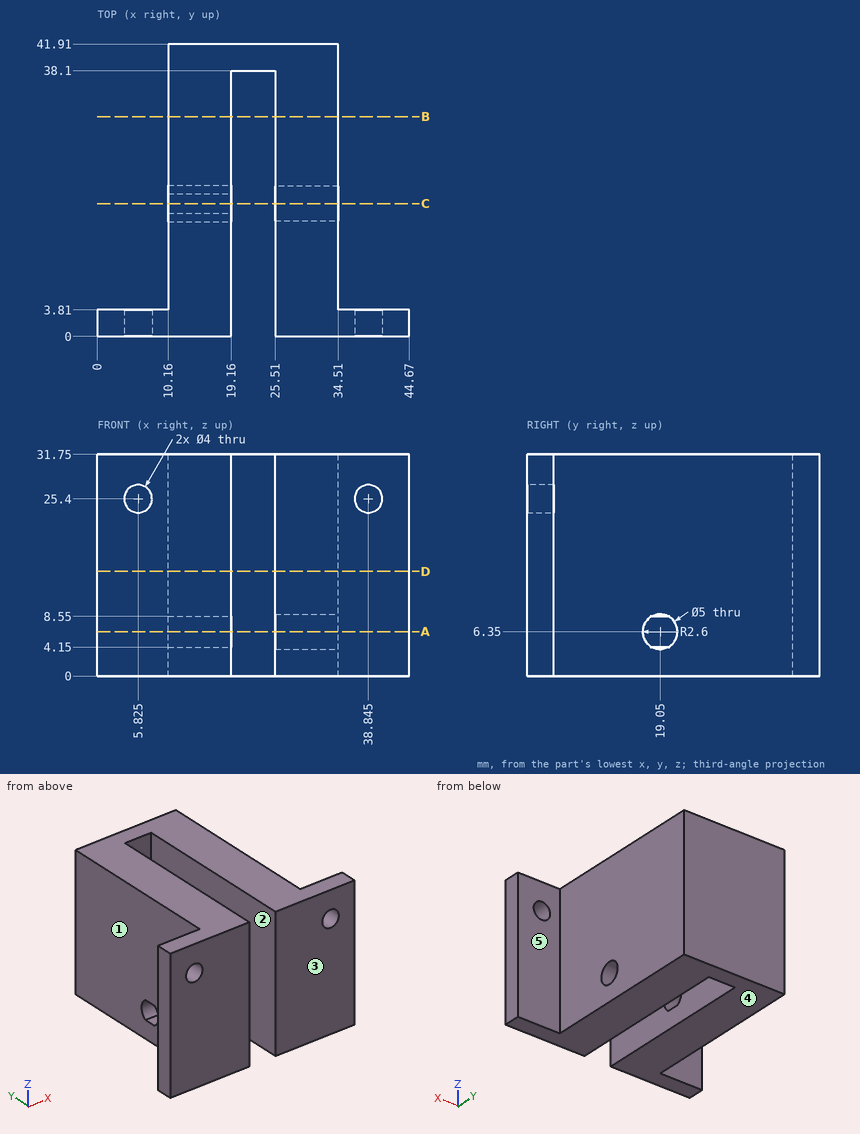
Check sheet for the drawn part. Datum: minimum x, y, z corner. Units: mm. A direction names the side the tool comes from. Round coordinates to 2 decimals unless told otherwise and drop trailing zeros. Loops run counter-clockwise (first coordinate to the right, second up) from the corner with the lowest first, then second, coordinate; pieces in that order, holes last. Notation, with made-up numbers: (2.5, 8) - (51.5, 8) arc R24 ccw to (51.5, 42) - close; hole circle Ø1 at (83.5, 16). An arc over 180 degrees is marked (long way). Write item = value, one per line. Start each with the question number.
1. Section check D-D on z = 15. Enter the section's corners in (x, y), then the cut area to 3 significant figures.
2. Section check C-C on y = 19.05. Enter the section's corners in (x, z).
3. Section check A-A on z = 6.35. Enter the section's corners in (x, y).
4. Set-up check for the marked faces 1, 2, 3, 4 and 5: record each of +Z, -Z, +X, -X, +Y, -Y from which the full face is reachable in a straight line by a thin tool's end or side.
5. Thickness scan on line 1 (X direction, y = 0.9, z = 25.4) (3 decimals); line 2 (X direction, y = 31, z = 17.5); line 3 (Y direction, x = 16, z = 6.5). Record the ranges inside material, lowest first.
6. Section check B-B on y = 31.5. Enter the section's corners in (x, z), then the cut area to 4 significant figures.
7. Depth check by flat-ended pin: pin 1 (12 mm diameter, centred on y = 10.5, z = 16, fed in from -X); pin 2 (5 mm diameter, centred on x = 22, z = 17, fed in from -Y); pin 3 (12 mm diameter, centred on x = 25, y = 25, fed in from -Z); pin 4 (3 mm diameter, centred on y = 14, z = 23.5, fed in from +X). Enter the tip coordinate at first touch or a pass-through.
Working result:
q1.outline = (0, 0) - (19.16, 0) - (19.16, 38.1) - (25.51, 38.1) - (25.51, 0) - (44.67, 0) - (44.67, 3.81) - (34.51, 3.81) - (34.51, 41.91) - (10.16, 41.91) - (10.16, 3.81) - (0, 3.81) - close
q1.area = 856 mm^2
q2.outline = (10.16, 0) - (19.16, 0) - (19.16, 4.15) - (10.16, 4.15) - close; (10.16, 8.55) - (19.16, 8.55) - (19.16, 31.75) - (10.16, 31.75) - close; (25.51, 0) - (34.51, 0) - (34.51, 3.85) - (25.51, 3.85) - close; (25.51, 8.85) - (34.51, 8.85) - (34.51, 31.75) - (25.51, 31.75) - close
q3.outline = (0, 0) - (19.16, 0) - (19.16, 16.45) - (10.16, 16.45) - (10.16, 3.81) - (0, 3.81) - close; (10.16, 21.65) - (19.16, 21.65) - (19.16, 38.1) - (25.51, 38.1) - (25.51, 21.55) - (34.51, 21.55) - (34.51, 41.91) - (10.16, 41.91) - close; (25.51, 0) - (44.67, 0) - (44.67, 3.81) - (34.51, 3.81) - (34.51, 16.55) - (25.51, 16.55) - close
q4.face_1 = +Z, -Z, -X, +Y
q4.face_2 = +Z, -Z, -Y
q4.face_3 = +Z, -Z, +X, -X, -Y
q4.face_4 = -Z, +X, -X, +Y, -Y
q4.face_5 = +Z, -Z, +X, +Y
q5.line_1 = 0 to 3.825, 7.825 to 19.16, 25.51 to 36.845, 40.845 to 44.67
q5.line_2 = 10.16 to 19.16, 25.51 to 34.51
q5.line_3 = 0 to 16.45, 21.65 to 41.91
q6.outline = (10.16, 0) - (19.16, 0) - (19.16, 31.75) - (10.16, 31.75) - close; (25.51, 0) - (34.51, 0) - (34.51, 31.75) - (25.51, 31.75) - close
q6.area = 571.5 mm^2
q7.pin_1 = 10.16
q7.pin_2 = 38.1
q7.pin_3 = 0
q7.pin_4 = 34.51
